Here's how the part is built. I have some questions about the finished solid (model axes, mm). A direction names the side the tool comes from. Round coordinates to 2 decimals unless told otherwise and drop trailing zeros. Loops run counter-clockwise (first coordinate to the right, second up) from the corner with the lowest first, then second, coordinate; pieces in that order, holes last. Notation, with made-up numbers: (86.5, 86) -> (125.5, 86) arc R17 cw to (125.5, 100) -> close; hole circle Ø2 at (-2, 54). An arc over 180 degrees is marked (long way). One line per item, written item: value. Start each with the question number.
```python
from build123d import *

# Parameters (mm, degrees)
F1_DEPTH = 25.4
F3_DEPTH = 25.4
F5_DEPTH = 25.4
F6_R     = 6.35
F7_DEPTH = 25.4
F8_R     = 6.35
F9_DEPTH = 25.4


with BuildPart() as f1:
    # F0 (on Front) → F1 (new body)
    with BuildSketch(Plane.XZ):
        Polygon((0, 50.8), (0, 0), (76.2, 0), (76.2, 14.440612), (25.4, 14.440612), (25.4, 50.8), align=None)
    extrude(amount=F1_DEPTH)

    # F2 (on face) → F3 (cut)
    with BuildSketch(Plane.YZ.offset(25.4)):
        with BuildLine():
            Line((-25.4, 50.8), (-25.4, 31.75))
            ThreePointArc((-25.4, 31.75), (-21.90426, 42.748523), (-12.7, 49.710512))
            ThreePointArc((-12.7, 49.710512), (-15.828607, 50.525653), (-19.05, 50.8))
            Line((-19.05, 50.8), (-25.4, 50.8))
        make_face()
        with BuildLine():
            ThreePointArc((-6.35, 50.8), (-9.571393, 50.525653), (-12.7, 49.710512))
            ThreePointArc((-12.7, 49.710512), (-3.49574, 42.748523), (0, 31.75))
            Line((0, 31.75), (0, 50.8))
            Line((0, 50.8), (-6.35, 50.8))
        make_face()
        with BuildLine():
            ThreePointArc((-19.05, 50.8), (-15.828607, 50.525653), (-12.7, 49.710512))
            ThreePointArc((-12.7, 49.710512), (-9.571393, 50.525653), (-6.35, 50.8))
            Line((-6.35, 50.8), (-19.05, 50.8))
        make_face()
    extrude(amount=-F3_DEPTH, mode=Mode.SUBTRACT)

    # F4 (on face) → F5 (cut)
    with BuildSketch(Plane.YZ.offset(25.4)):
        with BuildLine():
            ThreePointArc((-12.7, 49.710512), (-16.058904, 48.140232), (-19.05, 45.949032))
            Line((-19.05, 45.949032), (-19.05, 36.398523))
            ThreePointArc((-19.05, 36.398523), (-17.190128, 31.908395), (-12.7, 30.048523))
            ThreePointArc((-12.7, 30.048523), (-8.209872, 31.908395), (-6.35, 36.398523))
            Line((-6.35, 36.398523), (-6.35, 45.949032))
            ThreePointArc((-6.35, 45.949032), (-9.341096, 48.140232), (-12.7, 49.710512))
        make_face()
    extrude(amount=-F5_DEPTH, mode=Mode.SUBTRACT)

    # F6 (on face) → F7 (cut)
    with BuildSketch(Plane.XY.offset(14.440612)):
        with Locations((38.1, -12.59214)):
            Circle(F6_R)
        with Locations((63.5, -12.7)):
            Circle(F6_R)
    extrude(amount=-F7_DEPTH, mode=Mode.SUBTRACT)

    # F8 (on face) → F9 (cut)
    with BuildSketch(Plane.XY.offset(14.440612)):
        with Locations((38.1, -12.59214)):
            Circle(F8_R)
        with Locations((63.5, -12.7)):
            Circle(F8_R)
        with BuildLine():
            Line((76.2, 0), (69.85, 0))
            ThreePointArc((69.85, 0), (74.340128, -1.859872), (76.2, -6.35))
            Line((76.2, -6.35), (76.2, 0))
        make_face()
        with BuildLine():
            ThreePointArc((76.2, -19.05), (74.340128, -23.540128), (69.85, -25.4))
            Line((69.85, -25.4), (76.2, -25.4))
            Line((76.2, -25.4), (76.2, -19.05))
        make_face()
    extrude(amount=-F9_DEPTH, mode=Mode.SUBTRACT)


solid = f1.part
```
Q1. Will these pins go through, and if not, where does the flat tip stop? P1, Ø10.5, axis at x = 9, z = 39, coming from the +Y side; P2, Ø2, axis at y = -20, z = 28.5, coming from the +X side; P3, Ø3, axis at x = 12.5, z = 42, coming from the -Y side.
Q2. I want a section at D-D on z = 41.5. Please give me the cut outline in (x, y).
Q3. I want a section at B-B on y = -9.5. Please give me the cut outline in (x, z), plus the area to 3 significant figures.
Q4. I want a section at C-C on x = 22.5. Please give me the cut outline in (y, z), plus the area to 3 significant figures.
Q5. I want a section at A-A on x = 63.5. Please give me the cut outline in (y, z), plus the area to 3 significant figures.
Q6. If I drill on line 1 along Y through (x, z) = (63.5, 10.25); line 2 along Y through (x, z) = (38.1, 5); line 3 along X through (y, z) = (-20.75, 28.5), over which ranges is the centre line in solid material (lowest first)?
Q7. If we mould it in two halves opening along X, with no side actions, what happens to faces 1 (the cylindrical face through (74.29, -1.81, 7.32)), 2 (the cylindrical face through (31.756, -12.313, 7.321)), 3 (the flat face through (13, -6.35, 41))? For each: released by +X, released by -X, zero draft, split by the parting line, or undercut.
Q8. Which directions (+Z, -Z, +X, -X, +Y, -Y) give clear straight access to the entire face, cutting with the end or side of a thin tool? Please do faces 4 (the flat face through (0, -13, 18)), 5 (the flat face through (51, -13, 14.441)), 6 (the flat face through (13, -19.05, 41)).
Answers below:
1. P1: stops at y = -0.11
1. P2: stops at x = 25.4
1. P3: stops at y = -23.27
2. outline: (0, -22.72) -> (25.4, -22.72) -> (25.4, -19.05) -> (0, -19.05) -> close; (0, -6.35) -> (25.4, -6.35) -> (25.4, -2.68) -> (0, -2.68) -> close
3. outline: (0, 0) -> (32.55, 0) -> (32.55, 14.44) -> (25.4, 14.44) -> (25.4, 30.91) -> (0, 30.91) -> close; (43.65, 0) -> (58.02, 0) -> (58.02, 14.44) -> (43.65, 14.44) -> close; (68.98, 0) -> (76.2, 0) -> (76.2, 14.44) -> (68.98, 14.44) -> close
3. area: 1,200 mm^2
4. outline: (-25.4, 0) -> (0, 0) -> (0, 31.75) arc R19.05 ccw to (-6.35, 45.95) -> (-6.35, 36.4) arc R6.35 cw to (-19.05, 36.4) -> (-19.05, 45.95) arc R19.05 ccw to (-25.4, 31.75) -> close
4. area: 927 mm^2
5. outline: (-25.4, 0) -> (-19.05, 0) -> (-19.05, 14.44) -> (-25.4, 14.44) -> close; (-6.35, 0) -> (0, 0) -> (0, 14.44) -> (-6.35, 14.44) -> close
5. area: 183 mm^2
6. line 1: y = -25.4 to -19.05, -6.35 to 0
6. line 2: y = -25.4 to -18.94, -6.24 to 0
6. line 3: x = 0 to 25.4
7. face 1: released by +X
7. face 2: undercut
7. face 3: zero draft
8. face 4: +Z, -Z, -X, +Y, -Y
8. face 5: +Z, +X, +Y, -Y
8. face 6: +Z, +X, -X
